Geometry check sheet. Reference: drawing and pictorial views, mm from the part's lowest x, y, z. Round coordinates to 2 decimals unless told otherwise and drop trailing zeros. Loops run counter-clockwise (first coordinate to the right, second up) from the corner with the lowest first, then second, coordinate; pieces in that order, holes last. Notation, with made-up numbers: (-6, -35.75) - (7, -35.75) arc R17 ccw to (7, -18.75) - close; hole circle Ø1 at (71, 16). An arc over 180 degrees is marked (long way). Return JSON: item names as keys, results as strings.
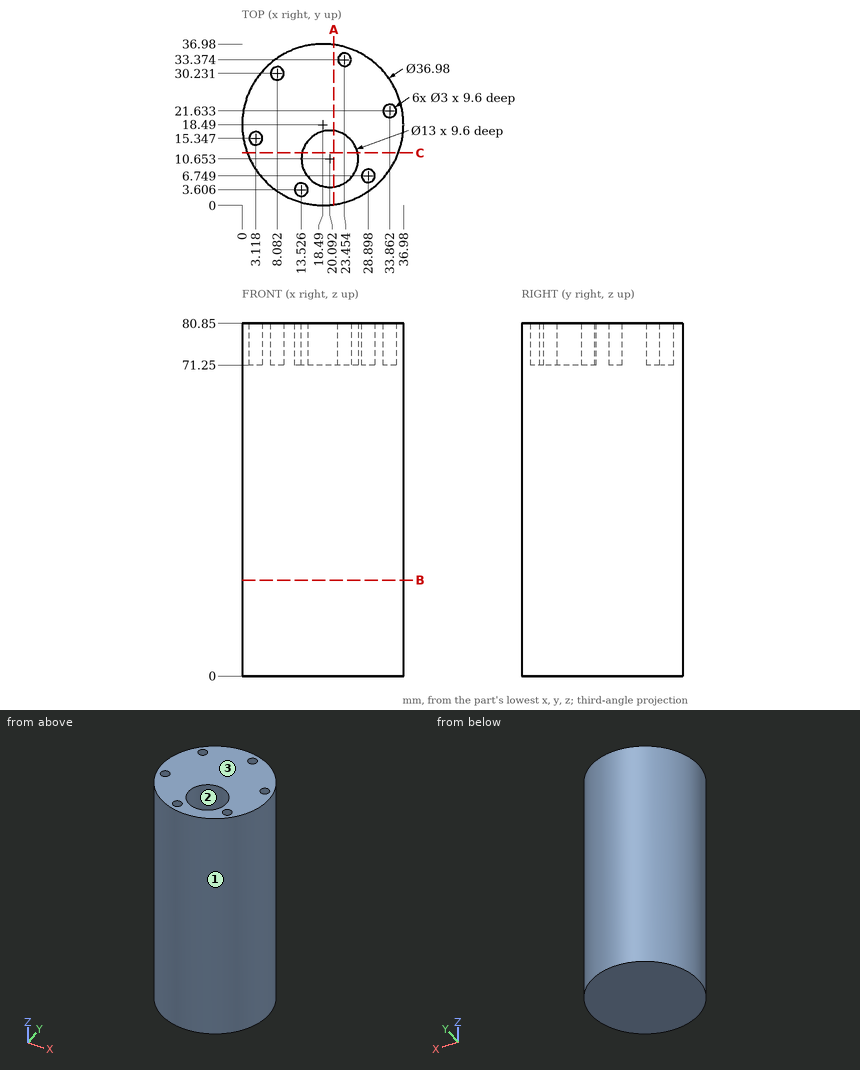
Q1. Scan lines: probe 1 along Z at (x, y) = (20.5, 16.5); probe 2 along Y at (x, z) = (24, 65); probe 3 along Y at (x, z) = (13, 74) (1 decimal). Record each from-to range of solid material in increasing order. Write a range as [from, to].
Answer key:
{"probe 1": "z = [0, 71.25]", "probe 2": "y = [0.84, 36.14]", "probe 3": "y = [0.8, 2.2], [5, 36.1]"}
Q2. Depth check by flat-ended pin: P1, Ø6, axis at y = 11.5, z = 15, coming from the +X side (1 decimal); P2, Ø3.5, axis at x = 8.08, y = 30.23, coming from the -Z side; P3, Ø0.9, axis at x = 13, y = 4, coming from the +Z side; P4, Ø4, axis at y = 8.5, z = 43, coming from the -X side (1 decimal). Enter the tip coordinate at first touch or a pass-through.
Answer key:
{"P1": "stops at x = 36.5", "P2": "stops at z = 0", "P3": "stops at z = 71.25", "P4": "stops at x = 1.8"}
Q3. Sectioned sample at A-A (x = 21). Enter the section's corners in (y, z), plus the area to 3 significant figures.
Answer key:
{"outline": "(0.17, 0) - (36.81, 0) - (36.81, 80.85) - (17.09, 80.85) - (17.09, 71.25) - (4.22, 71.25) - (4.22, 80.85) - (0.17, 80.85) - close", "area": "2,840 mm²"}
Q4. Draft check along Y on the marked faces 1, 2 and 3. Enter one of: released by +Y, released by -Y, zero draft, split by the parting line, or undercut.
Answer key:
{"face 1": "split by the parting line", "face 2": "undercut", "face 3": "zero draft"}
Q5. Sectioned sample at C-C (y = 12). Enter the section's corners in (x, z).
Answer key:
{"outline": "(1.18, 0) - (35.8, 0) - (35.8, 80.85) - (26.45, 80.85) - (26.45, 71.25) - (13.73, 71.25) - (13.73, 80.85) - (1.18, 80.85) - close"}
Q6. Sectioned sample at B-B (z = 22). Enter the section's corners in (x, y).
Answer key:
{"outline": "circle Ø36.98 at (18.49, 18.49)"}
